```python
from build123d import *

# Parameters (mm, degrees)
BOSS_EXTRUDE1_DEPTH = 2.54


with BuildPart() as part:
    # Sketch1 → Boss-Extrude1 (new body)
    with BuildSketch(Plane.XY):
        Polygon((-2.930050059, -104.509781075), (-3.314938219, -104.509781075), (-3.314938219, -110.859781075), (-3.314938219, -123.559781075), (-2.930050059, -123.559781075), (-2.930050059, -168.708281075), (38.709428475, -168.708281075), (38.709428475, -189.536281075), (105.397061781, -189.536281075), (66.517436481, -110.859781075), (47.485061781, -110.859781075), (47.485061781, -104.509781075), (47.485061781, -72.886781075), (47.485061781, -66.536781075), (66.517436481, -66.536781075), (105.397061781, 12.139718925), (38.709428475, 12.139718925), (38.709428475, -8.688281075), (-2.930050059, -8.688281075), (-2.930050059, -53.836781075), (-3.314938219, -53.836781075), (-3.314938219, -66.536781075), (-3.314938219, -72.886781075), (-2.930050059, -72.886781075), align=None)
        Polygon((4.868148885, -57.011781075), (6.70123599, -60.186781075), (4.868148885, -63.361781075), (1.201974676, -63.361781075), (-0.631112429, -60.186781075), (1.201974676, -57.011781075), align=None, mode=Mode.SUBTRACT)
        Polygon((45.622728689, -160.961281075), (43.789641585, -157.786281075), (40.123467375, -157.786281075), (38.290380271, -160.961281075), (40.123467375, -164.136281075), (43.789641585, -164.136281075), align=None, mode=Mode.SUBTRACT)
        Polygon((92.506998247, -183.186281075), (88.840824038, -183.186281075), (87.007736933, -180.011281075), (88.840824038, -176.836281075), (92.506998247, -176.836281075), (94.340085352, -180.011281075), align=None, mode=Mode.SUBTRACT)
        Polygon((88.840824038, -0.560281075), (87.007736933, 2.614718925), (88.840824038, 5.789718925), (92.506998247, 5.789718925), (94.340085352, 2.614718925), (92.506998247, -0.560281075), align=None, mode=Mode.SUBTRACT)
        Polygon((43.789641585, -13.260281075), (45.622728689, -16.435281075), (43.789641585, -19.610281075), (40.123467375, -19.610281075), (38.290380271, -16.435281075), (40.123467375, -13.260281075), align=None, mode=Mode.SUBTRACT)
        Polygon((1.201974676, -120.384781075), (4.868148885, -120.384781075), (6.70123599, -117.209781075), (4.868148885, -114.034781075), (1.201974676, -114.034781075), (-0.631112429, -117.209781075), align=None, mode=Mode.SUBTRACT)
    extrude(amount=BOSS_EXTRUDE1_DEPTH)


solid = part.part
```
Design review of the part built by this model. Coordinates are the model's own, in mm. Round coordinates to 2 decimals unless told otherwise and drop trailing zeros. Order: outer loops, then holes, each group sorted by start corner. A loop starts at its lowest first (then second) coordinate and runs counter-clockwise, first axis right, second up. Notation, with made-up numbers: (68.5, -18.5) - (93.5, -18.5) arc R14 ccw to (93.5, -3.5) - close; hole circle Ø8 at (67.5, 63). An arc over 180 degrees is marked (long way). Return JSON: item names as keys, results as strings.
Q1. Consider section C-C on y = -88.5. Write out the cut boundary in (x, z), plus the area to 3 significant figures.
Computed values:
{"outline": "(-2.93, 0) - (47.49, 0) - (47.49, 2.54) - (-2.93, 2.54) - close", "area": "128 mm2"}
Q2. The part is to be moulded in two halves that separate along Y. For faces 1 (the flat face through (38, -87, 0)), 2 (the flat face through (85.685, -27.749, 1.252)), 3 (the flat face through (86.23, -150.75, 1.25)), say which applies: pulls with the +Y half, pulls with the -Y half, needs draft (parallel to the pull), parting line crosses it, or undercut.
Computed values:
{"face 1": "needs draft", "face 2": "undercut", "face 3": "undercut"}
Q3. Consider section B-B on z = 1.5. Give the number of separate pieces and of enclosed holes in the cut face, plus the area to 3 significant figures.
Computed values:
{"separate pieces": "1", "enclosed holes": "6", "area": "14,300 mm2"}
Q4. Consider section A-A on x = 62. Write out the cut boundary in (y, z), plus the area to 3 significant figures.
Computed values:
{"outline": "(-189.54, 0) - (-110.86, 0) - (-110.86, 2.54) - (-189.54, 2.54) - close; (-66.54, 0) - (12.14, 0) - (12.14, 2.54) - (-66.54, 2.54) - close", "area": "400 mm2"}
Q5. For pin 1 Ø1.5 at (x, z) = (22, 2) entering from -Y; pin 2 Ø1.3 at (y, z) = (3.5, 1) entering from -X; pin 3 Ø1 at (y, z) = (-93.5, 2) entering from +X, all flat-tipped, find the tip position at first contact; note any pin that passes through.
Computed values:
{"pin 1": "stops at y = -168.71", "pin 2": "stops at x = 38.71", "pin 3": "stops at x = 47.49"}
Q6. Wall thickness on L1, parallel to Y at x = 48, z = 1.1; L2, parallel to Y at x = 16, z = 0.85; L3, parallel to Y at x = 39, z = 0.75: over which ranges is each line inside the solid? List them lowest first. Write a range as [from, to].
Computed values:
{"L1": "y = [-189.54, -110.86], [-66.54, 12.14]", "L2": "y = [-168.71, -8.69]", "L3": "y = [-189.54, -162.19], [-159.73, -17.66], [-15.21, 12.14]"}
Q7. Consider section D-D on x = 35. Write out the cut boundary in (y, z), plus the area to 3 significant figures.
Computed values:
{"outline": "(-168.71, 0) - (-8.69, 0) - (-8.69, 2.54) - (-168.71, 2.54) - close", "area": "406 mm2"}
